Geometry: final body of the model. Coordinates: model frame, mm. Face numbers are marked on the shaded views. Coordinates: 2 decimals unless noted, no trailing zeros. Write each loop counter-clockwise with the first axis right and the second up, starting at its lowest first coordinate (ties: lowest second). Pieces come first, ordered by that corner, then holes. Notation, with made-up numbers: (18.25, -32) - (57.25, -32) arc R12 ccw to (57.25, -9) - close; hole circle Ø7 at (-13.75, 60). An arc over 180 degrees is marked (long way). Answer as a JSON object with one key per item and string values. Group by question number.
Item 1: Section B-B on y = -31.75. Return loops of the section in (x, z) (3 decimals), and give its area (3 significant figures).
Item 2: Section A-A on x = 13.97. Return loops of the section in (y, z), and give its area (3 significant figures).
Item 3: First-contact query: pin 1 Ø6 at (x, y) = (-13.97, -31.75) entering from -Z; pin 2 Ø10 at (x, y) = (-2.5, -21.5) entering from -Z; pin 3 Ø2 at (x, z) = (13.97, -67.9) entering from +Y. Flat tips, straight axial feed; report the tip coordinate or a pass-through.
Item 4: Line query: line 1 along X through (y, z) = (-31.75, 4.1) (3 decimals); line 2 along Z through (x, y) = (13.97, -1.3); line 3 along X through (y, z) = (-19, -65.5) (3 decimals). Output: solid intervals per line, ascending. Write a range as from..to.
Item 5: Mould query, pull axis X, two halves, no side actions, for the marked faces 1, 2, 3 and 4. Classes: pulls with the +X half, pulls with the -X half, needs draft (parallel to the pull), parting line crosses it, or undercut.
Item 6: Section D-D on x = -0.5. Return loops of the section in (y, z), and give its area (3 significant figures).
Item 7: Section C-C on z = -61. Return loops of the section in (x, y) (3 decimals).
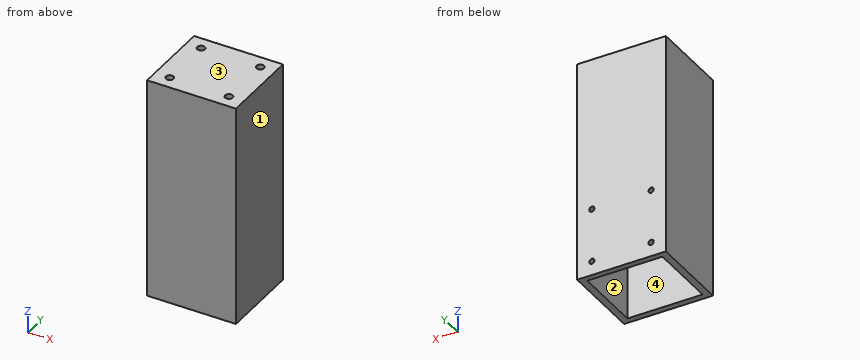
```python
from build123d import *

# Parameters (mm, degrees)
SKETCH3_W                                           = 20.955
SKETCH3_H                                           = 38.1
BOSS_EXTRUDE1_DEPTH                                 = 5
CSK_FOR_M3_COUNTERSUNK_FLAT_HEAD_SCREW1_D           = 3.6
CSK_FOR_M3_COUNTERSUNK_FLAT_HEAD_SCREW1_DEPTH       = 10
CSK_FOR_M3_COUNTERSUNK_FLAT_HEAD_SCREW1_CSINK_D     = 6.3
CSK_FOR_M3_COUNTERSUNK_FLAT_HEAD_SCREW1_CSINK_ANGLE = 90
CSK_FOR_M3_COUNTERSUNK_FLAT_HEAD_SCREW1_TIP         = 1.081549114
CSK_FOR_M3_COUNTERSUNK_FLAT_HEAD_SCREW2_D           = 3.6
CSK_FOR_M3_COUNTERSUNK_FLAT_HEAD_SCREW2_DEPTH       = 10
CSK_FOR_M3_COUNTERSUNK_FLAT_HEAD_SCREW2_CSINK_D     = 6.3
CSK_FOR_M3_COUNTERSUNK_FLAT_HEAD_SCREW2_CSINK_ANGLE = 90
CSK_FOR_M3_COUNTERSUNK_FLAT_HEAD_SCREW2_TIP         = 1.081549114
SKETCH12_W                                          = 41.91
SKETCH12_H                                          = 38.1
BOSS_EXTRUDE2_DEPTH                                 = 100
SKETCH15_W                                          = 35.458687416
SKETCH15_H                                          = 32.541680012
CUT_EXTRUDE4_DEPTH                                  = 100
M3_TAPPED_HOLE1_D                                   = 2.5
M3_TAPPED_HOLE1_DEPTH                               = 10
M3_TAPPED_HOLE1_TIP                                 = 0.751075774


with BuildPart() as part:
    # Sketch3 → Boss-Extrude1 (new body)
    with BuildSketch(Plane.XY):
        with Locations((10.4775, -19.05)):
            Rectangle(SKETCH3_W, SKETCH3_H)
        with Locations((-10.4775, -19.05)):
            Rectangle(SKETCH3_W, SKETCH3_H)
    extrude(amount=BOSS_EXTRUDE1_DEPTH)

    # CSK for M3 Countersunk Flat Head Screw1
    with Locations(Plane(origin=(0, 0, 0), x_dir=(1, 0, 0), z_dir=(0, 0, -1))):
        with Locations((-13.97, 6.35)):
            CounterSinkHole(CSK_FOR_M3_COUNTERSUNK_FLAT_HEAD_SCREW1_D / 2, CSK_FOR_M3_COUNTERSUNK_FLAT_HEAD_SCREW1_CSINK_D / 2, depth=CSK_FOR_M3_COUNTERSUNK_FLAT_HEAD_SCREW1_DEPTH, counter_sink_angle=CSK_FOR_M3_COUNTERSUNK_FLAT_HEAD_SCREW1_CSINK_ANGLE)
            with Locations((0, 0, -(CSK_FOR_M3_COUNTERSUNK_FLAT_HEAD_SCREW1_DEPTH + CSK_FOR_M3_COUNTERSUNK_FLAT_HEAD_SCREW1_TIP / 2))):  # 118° drill point
                Cone(0, CSK_FOR_M3_COUNTERSUNK_FLAT_HEAD_SCREW1_D / 2, CSK_FOR_M3_COUNTERSUNK_FLAT_HEAD_SCREW1_TIP, mode=Mode.SUBTRACT)

    # CSK for M3 Countersunk Flat Head Screw2
    with Locations(Plane(origin=(0, 0, 0), x_dir=(1, 0, 0), z_dir=(0, 0, -1))):
        with Locations((-13.97, 31.75), (-13.97, 6.35), (13.97, 6.35), (13.97, 31.75)):
            CounterSinkHole(CSK_FOR_M3_COUNTERSUNK_FLAT_HEAD_SCREW2_D / 2, CSK_FOR_M3_COUNTERSUNK_FLAT_HEAD_SCREW2_CSINK_D / 2, depth=CSK_FOR_M3_COUNTERSUNK_FLAT_HEAD_SCREW2_DEPTH, counter_sink_angle=CSK_FOR_M3_COUNTERSUNK_FLAT_HEAD_SCREW2_CSINK_ANGLE)
            with Locations((0, 0, -(CSK_FOR_M3_COUNTERSUNK_FLAT_HEAD_SCREW2_DEPTH + CSK_FOR_M3_COUNTERSUNK_FLAT_HEAD_SCREW2_TIP / 2))):  # 118° drill point
                Cone(0, CSK_FOR_M3_COUNTERSUNK_FLAT_HEAD_SCREW2_D / 2, CSK_FOR_M3_COUNTERSUNK_FLAT_HEAD_SCREW2_TIP, mode=Mode.SUBTRACT)

    # Sketch12 → Boss-Extrude2 (add)
    with BuildSketch(Plane(origin=(0, 0, 0), x_dir=(-1, 0, 0), z_dir=(0, 0, -1))):
        with Locations((0, -19.05)):
            Rectangle(SKETCH12_W, SKETCH12_H)
    extrude(amount=BOSS_EXTRUDE2_DEPTH)

    # Sketch15 → Cut-Extrude4 (cut)
    with BuildSketch(Plane(origin=(0, 0, -100), x_dir=(-1, 0, 0), z_dir=(0, 0, -1))):
        with Locations((0, -18.974233574)):
            Rectangle(SKETCH15_W, SKETCH15_H)
    extrude(amount=-CUT_EXTRUDE4_DEPTH, mode=Mode.SUBTRACT)

    # M3 Tapped Hole1
    with Locations(Plane(origin=(0, 0, 0), x_dir=(1, 0, 0), z_dir=(0, 1, 0))):
        with Locations((-13.97, 93.295610143), (-13.97, 67.895610143), (13.97, 67.895610143), (13.97, 93.295610143)):
            Hole(M3_TAPPED_HOLE1_D / 2, depth=M3_TAPPED_HOLE1_DEPTH)
            with Locations((0, 0, -(M3_TAPPED_HOLE1_DEPTH + M3_TAPPED_HOLE1_TIP / 2))):  # 118° drill point
                Cone(0, M3_TAPPED_HOLE1_D / 2, M3_TAPPED_HOLE1_TIP, mode=Mode.SUBTRACT)


solid = part.part
```
Checks:
{
 "1": {"outline": "(-20.955, -100) - (-17.729, -100) - (-17.729, 0) - (-17.12, 0) - (-15.77, 1.35) - (-15.77, 5) - (-20.955, 5) - close; (-12.17, 1.35) - (-10.82, 0) - (10.82, 0) - (12.17, 1.35) - (12.17, 5) - (-12.17, 5) - close; (15.77, 1.35) - (17.12, 0) - (17.729, 0) - (17.729, -100) - (20.955, -100) - (20.955, 5) - (15.77, 5) - close", "area": "815 mm^2"},
 "2": {"outline": "(-38.1, -100) - (-35.25, -100) - (-35.25, 0) - (-34.9, 0) - (-33.55, 1.35) - (-33.55, 5) - (-38.1, 5) - close; (-29.95, 1.35) - (-28.6, 0) - (-9.5, 0) - (-8.15, 1.35) - (-8.15, 5) - (-29.95, 5) - close; (-4.55, 1.35) - (-3.2, 0) - (-2.7, 0) - (-2.7, -66.65) - (0, -66.65) - (0, 5) - (-4.55, 5) - close; (-2.7, -100) - (0, -100) - (0, -94.55) - (-2.7, -94.55) - close; (-2.7, -92.05) - (0, -92.05) - (0, -69.15) - (-2.7, -69.15) - close", "area": "693 mm^2"},
 "3": {"pin 1": "z = 0.15", "pin 2": "z = 0", "pin 3": "y = -35.25"},
 "4": {"line 1": "-20.955..-15.77, -12.17..12.17, 15.77..20.955", "line 2": "-100..-94.55, -92.05..-69.15, -66.65..5", "line 3": "-20.955..-17.729, 17.729..20.955"},
 "5": {"face 1": "pulls with the +X half", "face 2": "undercut", "face 3": "needs draft", "face 4": "undercut"},
 "6": {"outline": "(-38.1, -100) - (-35.25, -100) - (-35.25, 0) - (-2.7, 0) - (-2.7, -100) - (0, -100) - (0, 5) - (-38.1, 5) - close", "area": "746 mm^2"},
 "7": {"outline": "(-20.955, -38.1) - (20.955, -38.1) - (20.955, 0) - (-20.955, 0) - close; hole (-17.729, -35.245) - (17.729, -35.245) - (17.729, -2.703) - (-17.729, -2.703) - close"}
}
